Verification items for the finished model (mm, model axes). Face numbers are marked on the shaded views. A direction names the side the tool comes from. Give positions to 0.01 mm unless a question says otherwise; leave off trailing zeros. Order: outer loops, then holes, each group sorted by start corner. A loop starts at its lowest first (then second) coordinate and runs counter-clockwise, first axis right, second up.
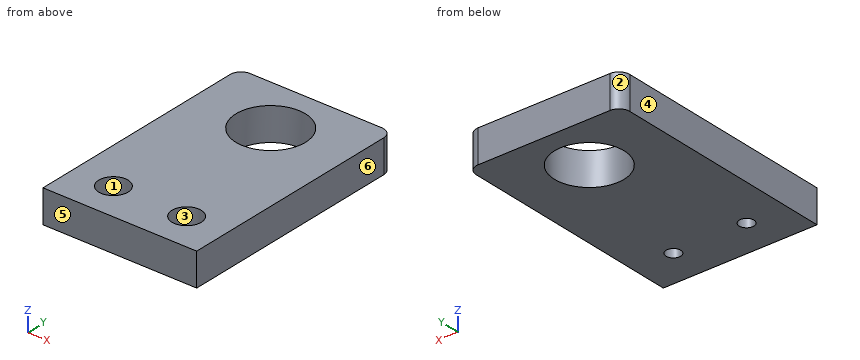
from build123d import *

# Parameters (mm, degrees)
CROQUIS1_R              = 9.5
CROQUIS1_R_2            = 2
SALIENTE_EXTRUIR1_DEPTH = 9
CROQUIS2_R              = 4
CORTAR_EXTRUIR1_DEPTH   = 4.5


with BuildPart() as part:
    # Croquis1 → Saliente-Extruir1 (new body)
    with BuildSketch(Plane.XY):
        with BuildLine():
            Line((-18, 32.5), (18, 32.5))
            ThreePointArc((18, 32.5), (20.121320344, 31.621320344), (21, 29.5))
            Line((21, 29.5), (21, -32.5))
            Line((21, -32.5), (-21, -32.5))
            Line((-21, -32.5), (-21, 29.5))
            ThreePointArc((-21, 29.5), (-20.121320344, 31.621320344), (-18, 32.5))
        make_face()
        with Locations((0, 17.5)):
            Circle(CROQUIS1_R, mode=Mode.SUBTRACT)
        with Locations((10, -22.5)):
            Circle(CROQUIS1_R_2, mode=Mode.SUBTRACT)
        with Locations((-10, -22.5)):
            Circle(CROQUIS1_R_2, mode=Mode.SUBTRACT)
    extrude(amount=SALIENTE_EXTRUIR1_DEPTH)

    # Croquis2 → Cortar-Extruir1 (cut)
    with BuildSketch(Plane.XY.offset(9)):
        with Locations((-10, -22.5)):
            Circle(CROQUIS2_R)
        with Locations((10, -22.5)):
            Circle(CROQUIS2_R)
    extrude(amount=-CORTAR_EXTRUIR1_DEPTH, mode=Mode.SUBTRACT)


solid = part.part
(1) Section check C-C, the plane x = 0. Enter the section's corners in (y, z).
Solved:
outline: (-32.5, 0) - (8, 0) - (8, 9) - (-32.5, 9) - close; (27, 0) - (32.5, 0) - (32.5, 9) - (27, 9) - close
(2) Set-up check for the marked faces 1 and 2: record each of +Z, -Z, +X, -X, +Y, -Y from which the full face is reachable in a straight line by a thin tool's end or side.
Solved:
face 1: +Z
face 2: +Z, -Z, -X, +Y
(3) Section check B-B, the plane z = 3. Enter the section's corners in (x, y).
Solved:
outline: (-21, -32.5) - (21, -32.5) - (21, 29.5) arc R3 ccw to (18, 32.5) - (-18, 32.5) arc R3 ccw to (-21, 29.5) - close; hole circle Ø4 at (-10, -22.5); hole circle Ø19 at (0, 17.5); hole circle Ø4 at (10, -22.5)
(4) Section check D-D, the plane y = -22.5. Enter the section's corners in (x, z), then the cut area to 3 significant figures.
Solved:
outline: (-21, 0) - (-12, 0) - (-12, 4.5) - (-14, 4.5) - (-14, 9) - (-21, 9) - close; (-8, 0) - (8, 0) - (8, 4.5) - (6, 4.5) - (6, 9) - (-6, 9) - (-6, 4.5) - (-8, 4.5) - close; (12, 0) - (21, 0) - (21, 9) - (14, 9) - (14, 4.5) - (12, 4.5) - close
area: 270 mm2
(5) Section check A-A, the plane y = 17.5. Enter the section's corners in (x, z).
Solved:
outline: (-21, 0) - (-9.5, 0) - (-9.5, 9) - (-21, 9) - close; (9.5, 0) - (21, 0) - (21, 9) - (9.5, 9) - close
(6) Go/stop test with flat-tipped pins: pin 1 (7 mm diameter, centred on x = -10, y = -22.5, fed in from +Z); pin 2 (11.5 mm diameter, centred on x = 0, y = 17.5, fed in from +Z). Record where each tip stops, or that it passes through.
Solved:
pin 1: stops at z = 4.5
pin 2: passes through
(7) Scan lines: line 1 (X direction, y = -22.5, z = 1.35); line 2 (Y direction, x = -10, z = 2.95); line 3 (Y direction, x = 0.5, z = 8.5). Record each from-to range of solid material in increasing order.
Solved:
line 1: x = -21 to -12, -8 to 8, 12 to 21
line 2: y = -32.5 to -24.5, -20.5 to 32.5
line 3: y = -32.5 to 8.01, 26.99 to 32.5
(8) Release check for a two-part mould opening along X. For the marked faces 3, 4, 5 and 6 record: pulls with the +X half, pulls with the -X half, needs draft (parallel to the pull), parting line crosses it, or undercut.
Solved:
face 3: undercut
face 4: pulls with the -X half
face 5: needs draft
face 6: pulls with the +X half
